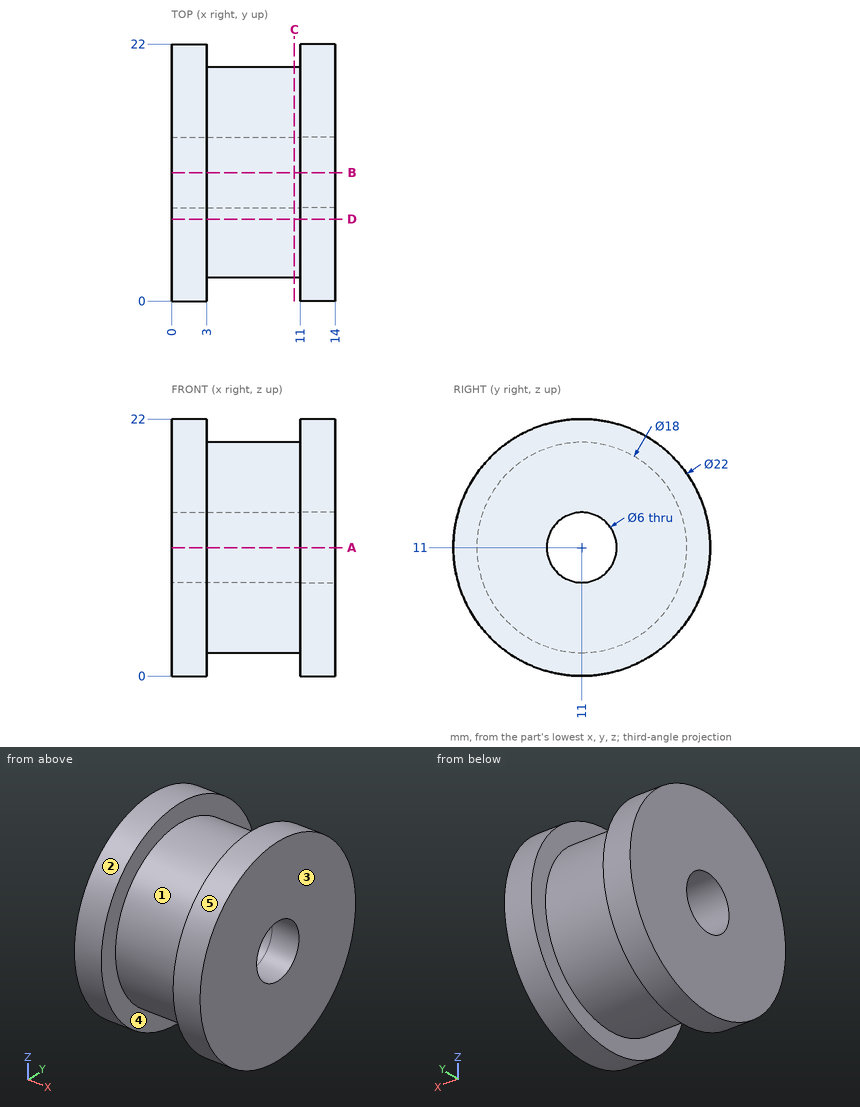
Check sheet for the drawn part. Datum: minimum x, y, z corner. Units: mm. A direction names the side the tool comes from. Give positions to 0.01 mm unless a question says otherwise; leave off trailing zeros. Loops run counter-clockwise (first coordinate to the right, second up) from the corner with the lowest first, then second, coordinate; pieces in that order, holes last. Notation, with made-up numbers: M -32.75,-21 L 9.25,-21 A29 cw 9.25,11 Z; hole C 85,-8.75 d1. An arc over 180 degrees is marked long. Answer as CSV lines item,"result".
Item 1: Sectioned sample at C-C, the plane x = 10.5. Enter the section's corners in (y, z), then the cut area to 3 significant figures.
Reply:
outline,"C 11,11 d18; hole C 11,11 d6"
area,"226 mm^2"
Item 2: Draft check along X on the marked faces 1, 2 and 3. Enter one of: pulls with the +X half, pulls with the -X half, needs draft (parallel to the pull), parting line crosses it, or undercut.
Reply:
face 1,"undercut"
face 2,"needs draft"
face 3,"pulls with the +X half"
Item 3: Sectioned sample at D-D, the plane y = 7. Enter the section's corners in (x, z), then the cut area to 3 significant figures.
Reply:
outline,"M 0,0.75 L 3,0.75 L 3,2.94 L 11,2.94 L 11,0.75 L 14,0.75 L 14,21.25 L 11,21.25 L 11,19.06 L 3,19.06 L 3,21.25 L 0,21.25 Z"
area,"252 mm^2"
Item 4: Sectioned sample at A-A, the plane z = 11. Enter the section's corners in (x, y), then the cut area to 3 significant figures.
Reply:
outline,"M 0,0 L 3,0 L 3,2 L 11,2 L 11,0 L 14,0 L 14,8 L 0,8 Z; M 0,14 L 14,14 L 14,22 L 11,22 L 11,20 L 3,20 L 3,22 L 0,22 Z"
area,"192 mm^2"
Item 5: Set-up check for the marked faces 4 and 5: record each of +Z, -Z, +X, -X, +Y, -Y from which the full face is reachable in a straight line by a thin tool's end or side.
Reply:
face 4,"none"
face 5,"+X, -X"
Item 6: Depth check by flat-ended pin: pin 1 Ø3 at (x, y) = (7, 2.5) entering from +Z; pin 2 Ø2 at (y, z) = (6, 10) entering from -X; pin 3 Ø5 at (x, z) = (7, 7.5) entering from +Y; pin 4 Ø1 at (x, y) = (9, 6.5) entering from -Z. Enter the tip coordinate at first touch or a pass-through.
Reply:
pin 1,"z = 16.66"
pin 2,"x = 0"
pin 3,"y = 19.94"
pin 4,"z = 2.94"
Item 7: Scan lines: L1, parallel to Y at x = 13.1, z = 11; L2, parallel to Y at x = 8.5, z = 11; L3, parallel to X at y = 10.75, z = 1.75. Record each from-to range of solid material in increasing order.
Reply:
L1,"0 to 8, 14 to 22"
L2,"2 to 8, 14 to 20"
L3,"0 to 3, 11 to 14"
